The model under review builds one solid part; all positions refer to its coordinate system, in mm. Coordinates: 2 decimals unless noted, no trailing zeros. Order: outer loops, then holes, each group sorted by start corner. A loop starts at its lowest first (then second) coordinate and runs counter-clockwise, first axis right, second up. Notation, with made-up numbers: (-14, 69) -> (44, 69) arc R20 ccw to (44, 85) -> close; hole circle Ø1 at (78.5, -39). An arc over 180 degrees is marked (long way). Answer as CSV lines item,"result". Start each with the question number.
from build123d import *

# Parameters (mm, degrees)
BOSS_EXTRUDE1_START     = -25
BOSS_EXTRUDE1_DEPTH     = 50
CUT_EXTRUDE1_DEPTH      = 341.53226913
CUT_EXTRUDE1_DEPTH_BACK = 341.53226913
CUT_EXTRUDE2_DEPTH      = 341.286795308
CUT_EXTRUDE2_DEPTH_BACK = 341.286795308
SKETCH4_R               = 20


# Read off the part's stored shape, not the designer's step: Boss-Extrude1
with BuildPart() as part:
    # Boss-Extrude1 outline → Boss-Extrude1 (new body)
    with BuildSketch(Plane.XY.offset(BOSS_EXTRUDE1_START)):
        with BuildLine():
            Line((175, 0), (215.218833807, 40.218833807))
            ThreePointArc((215.218833807, 40.218833807), (226.057471223, 56.440000887), (229.863494748, 75.574172084))
            add(Edge.make_bspline(
                [(229.863494748, 75.574172084), (229.863497015, 220.574172084), (130.657195822, 208), (130.657198498, 108), (160, 250), (60, 250)],
                knots=[0, 0, 0, 0, 0, 0, 1, 1, 1, 1, 1, 1], degree=5))
            Line((60, 250), (-60, 250))
            add(Edge.make_bspline(
                [(-60, 250), (-160, 250), (-130.657198498, 108), (-130.657195822, 208), (-229.863497015, 220.574172084), (-229.863494748, 75.574172084)],
                knots=[0, 0, 0, 0, 0, 0, 1, 1, 1, 1, 1, 1], degree=5))
            ThreePointArc((-229.863494748, 75.574172084), (-226.057471223, 56.440000887), (-215.218833807, 40.218833807))
            Line((-215.218833807, 40.218833807), (-175, 0))
            Line((-175, 0), (175, 0))
        make_face()
    extrude(amount=BOSS_EXTRUDE1_DEPTH)

    # Sketch2 → Cut-Extrude1 (cut, two sides: drawn at the far end of the back side and taken through both)
    with BuildSketch(Plane(origin=(0, 0, 0), x_dir=(0, 0, -1), z_dir=(1, 0, 0)).offset(-CUT_EXTRUDE1_DEPTH_BACK)):
        Polygon((23.039732542, -10), (-12.506441807, 260), (35, 260), (35, -10), align=None)
        Polygon((-23.039732542, 260), (12.506441807, -10), (-35, -10), (-35, 260), align=None)
    extrude(amount=CUT_EXTRUDE1_DEPTH + CUT_EXTRUDE1_DEPTH_BACK, mode=Mode.SUBTRACT)

    # Sketch4 → Cut-Extrude2 (cut, two sides: drawn at the far end of the back side and taken through both)
    with BuildSketch(Plane(origin=(0, 2.811189919, -21.353107392), x_dir=(-1, 0, 0), z_dir=(0, 0.13052619222005532, -0.99144486137381)).offset(-CUT_EXTRUDE2_DEPTH_BACK)):
        with Locations(Location((0, 124.321792579, 0), (0, 0, 90))):
            Circle(SKETCH4_R)
    extrude(amount=CUT_EXTRUDE2_DEPTH + CUT_EXTRUDE2_DEPTH_BACK, mode=Mode.SUBTRACT)


solid = part.part
1) Consider section A-A (x = -51.5). Give the boundary of the cut face in (y, z), plus the area to 3 significant figures.
2) Insertion check: pin 1 Ø1.5 at (x, y) = (46.5, 201) entering from -Z; pin 2 Ø6 at (x, y) = (128, 185.5) entering from +Z; pin 3 Ø4 at (x, y) = (-127, 122) entering from +Z (3 decimals); pin 4 Ø10 at (y, z) = (148.5, 16) entering from +X. Each pin has a flat end and moves straight along its axis. Give the tip position at first contact, or say it passes through.
3) Consider section B-B (y = 33.5). Give the boundary of the cut face in (x, z).
4) Wall thickness on L1, parallel to Z at x = 63.5, y = 18; L2, parallel to Z at x = 52, y = 77.5; L3, parallel to X at y = 65, z = -8: over which ranges is each line inside the solid? List them lowest first. Write a range as [from, to].
5) Mouldability with a two-part tool opening along Y and no side actions: class faces 1 (the face through (-7.66, 143.695, 2.535)), 2 (the face through (1, 250, 16)), 3 (the face through (195, 20, -14)) as released by +Y, released by -Y, zero draft, split by the parting line, or undercut.
Result:
1,outline,"(0, -21.72) -> (250, 11.19) -> (250, 21.72) -> (0, -11.19) -> close"
1,area,"2,630 mm2"
2,pin 1,"z = 4.64"
2,pin 2,"z = 13.63"
2,pin 3,"z = 5.135"
2,pin 4,"through"
3,outline,"(-208.5, -17.31) -> (208.5, -17.31) -> (208.5, -6.78) -> (-208.5, -6.78) -> close"
4,L1,"[-19.35, -8.82]"
4,L2,"[-11.52, -0.99]"
4,L3,"[-228.73, 228.73]"
5,face 1,"undercut"
5,face 2,"released by +Y"
5,face 3,"released by -Y"
